Geometry check sheet. Reference: the model listing, model coordinates, mm. Face numbers are marked on the shaded views. Round coordinates to 2 decimals unless told otherwise and drop trailing zeros. Order: outer loops, then holes, each group sorted by start corner. A loop starts at its lowest first (then second) coordinate and runs counter-clockwise, first axis right, second up. Notation, with made-up numbers: (9.25, 58) -> (68.25, 58) arc R30 cw to (68.25, 89) -> close; hole circle Ø6 at (77.25, 66). An arc over 180 degrees is marked (long way). Answer as a JSON object with one key per item and string values. Group by question number.
from build123d import *

# Parameters (mm, degrees)
F0_R     = 22.225
F0_R_2   = 19.685
F1_DEPTH = 304.8
F4_R     = 9.525
F7_D     = 5.4102
F7_DEPTH = 19.05
F7_TIP   = 1.6253880605
F8_R     = 1.5875


with BuildPart() as f1:
    # F0 (on Top) → F1 (new body)
    with BuildSketch(Plane.XY):
        Circle(F0_R)
        Circle(F0_R_2, mode=Mode.SUBTRACT)
    extrude(amount=F1_DEPTH)

    # F4 (on line) → F5 (join, up to the next surface of F1)
    with BuildSketch(Plane(origin=(-60.325, 0, 0), x_dir=(0, -1, 0), z_dir=(-1, 0, 0))):
        with Locations((0, 63.5)):
            Circle(F4_R)
    extrude(until=Until.NEXT, dir=(1, 0, 0))

    # F7
    with Locations(Plane(origin=(-60.325, 0, 0), x_dir=(0, -1, 0), z_dir=(-1, 0, 0))):
        with Locations((0, 63.5)):
            Hole(F7_D / 2, depth=F7_DEPTH)
            with Locations((0, 0, -(F7_DEPTH + F7_TIP / 2))):  # 118° drill point
                Cone(0, F7_D / 2, F7_TIP, mode=Mode.SUBTRACT)

    # F8
    f8_edges = [f1.edges().sort_by_distance(p)[0] for p in [
        (-60.325, 9.525, 63.5),
    ]]
    fillet(f8_edges, radius=F8_R)


solid = f1.part
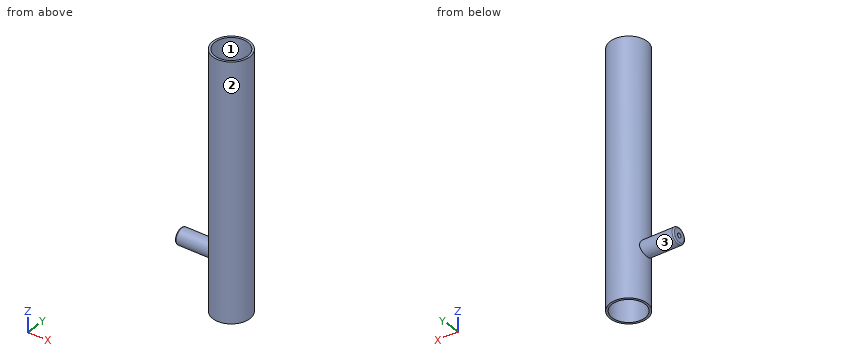
Item 1: Thickness scan on L1, parallel to Z at x = -45.75, y = 0 (3 decimals); L2, parallel to Y at x = 0, z = 94.5 (3 decimals); L3, parallel to Y at x = -47, z = 63.5 (3 decimals). Record the ranges inside material, lowest first.
Item 2: Sectioned sample at A-A, the plane x = 0. Enter the section's corners in (y, z) (3 decimals).
Item 3: Depth check by flat-ended pin: pin 1 Ø10 at (x, y) = (11, 10.5) entering from +Z; pin 2 Ø3 at (y, z) = (-9, 272) entering from +X; pin 3 Ø1.5 at (y, z) = (13, 197) entering from -X; pin 4 Ø4.5 at (y, z) = (0, 63.5) entering from -X. Enter the tip coordinate at first touch or a pass-through.
Item 4: Mould release check, pull along X, two halves, no side actions. Record for the marked faces 1, 2 and 3: pulls with the +X half, pulls with the -X half, needs draft (parallel to the pull), parting line crosses it, or undercut.
Item 5: Sectioned sample at B-B, the plane y = -17. Enter the section's corners in (x, z), then the cut area to 3 significant figures.
Item 6: Sectioned sample at C-C, the plane x = -46. Enter the section's corners in (y, z) (3 decimals).
Result:
{
 "1": {"L1": "z = 53.975 to 60.795, 66.205 to 73.025", "L2": "y = -22.225 to -19.685, 19.685 to 22.225", "L3": "y = -9.525 to -2.705, 2.705 to 9.525"},
 "2": {"outline": "(-22.225, 0) -> (-19.685, 0) -> (-19.685, 304.8) -> (-22.225, 304.8) -> close; (19.685, 0) -> (22.225, 0) -> (22.225, 304.8) -> (19.685, 304.8) -> close"},
 "3": {"pin 1": "stops at z = 304.8", "pin 2": "stops at x = 20.92", "pin 3": "stops at x = -18.54", "pin 4": "stops at x = -41"},
 "4": {"face 1": "undercut", "face 2": "parting line crosses it", "face 3": "needs draft"},
 "5": {"outline": "(-14.32, 0) -> (-9.92, 0) -> (-9.92, 304.8) -> (-14.32, 304.8) -> close; (9.92, 0) -> (14.32, 0) -> (14.32, 304.8) -> (9.92, 304.8) -> close", "area": "2,680 mm2"},
 "6": {"outline": "circle Ø19.05 at (0, 63.5); hole circle Ø5.41 at (0, 63.5)"}
}
